from build123d import *

# Parameters (mm, degrees)
F1_DEPTH    = 25.4
F2_R        = 1.27
F2_R_2      = 0.8255
F3_DEPTH    = 7.112
F3_FACE_R   = 1.27
F3_FACE_R_2 = 0.8255
F4_DEPTH    = 2.54


with BuildPart() as f1:
    # F0 (on Front) → F1 (new body)
    with BuildSketch(Plane.XZ):
        with BuildLine():
            Line((-6.35, 0), (0, 0))
            Line((0, 0), (0, 0.762))
            Line((0, 0.762), (-5.334, 0.762))
            ThreePointArc((-5.334, 0.762), (-5.963593, 7.744297), (0, 11.43))
            Line((0, 11.43), (0, 12.7))
            ThreePointArc((0, 12.7), (-7.099516, 8.312258), (-6.35, 0))
        make_face()
    extrude(amount=F1_DEPTH)

    # F2 (on Right) → F3 (join)
    with BuildSketch(Plane.YZ):
        with Locations((-21.872345, 3.302)):
            Circle(F2_R)
        with Locations((-21.872345, 3.302)):
            Circle(F2_R_2, mode=Mode.SUBTRACT)
    extrude(amount=-F3_DEPTH)

    # F3_face (on face) → F4 (join)
    with BuildSketch(Plane(origin=(0, -21.872345, 3.302), x_dir=(0, 1, 0), z_dir=(1, 0, 0))):
        Circle(F3_FACE_R)
        Circle(F3_FACE_R_2, mode=Mode.SUBTRACT)
    extrude(amount=F4_DEPTH)


solid = f1.part
Design review of the part built by this model. Coordinates are the model's own, in mm. A direction names the side the tool comes from. Coordinates: 2 decimals unless noted, no trailing zeros. Loops run counter-clockwise (first coordinate to the right, second up) from the corner with the lowest first, then second, coordinate; pieces in that order, holes last. Notation, with made-up numbers: (-31, 24.5) -> (-8, 24.5) arc R20 ccw to (-8, 37.5) -> close; hole circle Ø5 at (83.5, -26). An arc over 180 degrees is marked (long way). Use a Markdown table: item, result. Add a question column.
Item 1: We need section D-D, the plane z = 6.5. Write out the cut boundary in (x, y) (3 decimals), and give its area (3 significant figures).
Item 2: We need section A-A, the plane x = -3.5. Write out the cut boundary in (y, z), and give its area (3 significant figures).
Item 3: The part is to be moulded in two halves that separate along Z. For faces 3 (the flat face through (-6.34, 0, 7.32)), 4 (the flat face through (-3, -13, 0)), 5 (the cylindrical face through (-7.044, -12.522, 8.422)), 6 (the flat face through (-3, -13, 0.762)), say which applies: +Z half, -Z half, draft (parallel to the pull), parting line (faces both ways), or undercut.
Item 4: Wall thickness on L1, parallel to Y at x = 0, z = 3.25; L2, parallel to Z at x = -5.5, y = -2.75; L3, parallel to Z at x = -4, y = -12.5: over which ranges is each line inside the solid? List them lowest first. Write a range as from..to.
Item 5: We need section C-C, the plane x = -1.5. Write out the cut boundary in (y, z), and give its area (3 significant figures).
Item 6: Machinability: for faces 1 (the cylindrical face through (-2.13, -22.04, 4.56)), 2 (the flat face through (-6.34, -25.4, 7.32)), which of the approach directions +Z, -Z, +X, -X, +Y, -Y give a long, thin tool a straight path to every point of the face, cutting with its end or side? Answer none if there is none.
Item 7: Clearance check with flat-ended pins moving along their axes: P1, Ø1.5, axis at y = -20, z = 9, coming from the -X side; P2, Ø6, axis at y = -9, z = 2, coming from the +X side; P3, Ø1.9, axis at y = -21.87, z = 3.3, coming from the -X side. State where each tip first meets the part, or that it passes through.
Numbers:
| question | item | result |
|---|---|---|
| 1 | outline | (-7.745, -25.4) -> (-6.437, -25.4) -> (-6.437, 0) -> (-7.745, 0) -> close |
| 1 | area | 33.2 mm^2 |
| 2 | outline | (-25.4, 0) -> (0, 0) -> (0, 0.76) -> (-25.4, 0.76) -> close; (-25.4, 10.44) -> (0, 10.44) -> (0, 11.89) -> (-25.4, 11.89) -> close; circle Ø2.54 at (-21.87, 3.3); hole circle Ø1.65 at (-21.87, 3.3) |
| 2 | area | 59.1 mm^2 |
| 3 | face 3 | draft |
| 3 | face 4 | -Z half |
| 3 | face 5 | parting line |
| 3 | face 6 | undercut |
| 4 | L1 | y = -23.14..-22.7, -21.05..-20.6 |
| 4 | L2 | z = 0..0.99, 8.53..10.49 |
| 4 | L3 | z = 0..0.76, 10.1..11.62 |
| 5 | outline | (-25.4, 0) -> (0, 0) -> (0, 0.76) -> (-25.4, 0.76) -> close; (-25.4, 11.26) -> (0, 11.26) -> (0, 12.56) -> (-25.4, 12.56) -> close; circle Ø2.54 at (-21.87, 3.3); hole circle Ø1.65 at (-21.87, 3.3) |
| 5 | area | 55.2 mm^2 |
| 6 | face 1 | +X |
| 6 | face 2 | +Z, -Z, +X, -X, -Y |
| 7 | P1 | stops at x = -7.13 |
| 7 | P2 | stops at x = 0 |
| 7 | P3 | stops at x = -7.92 |
